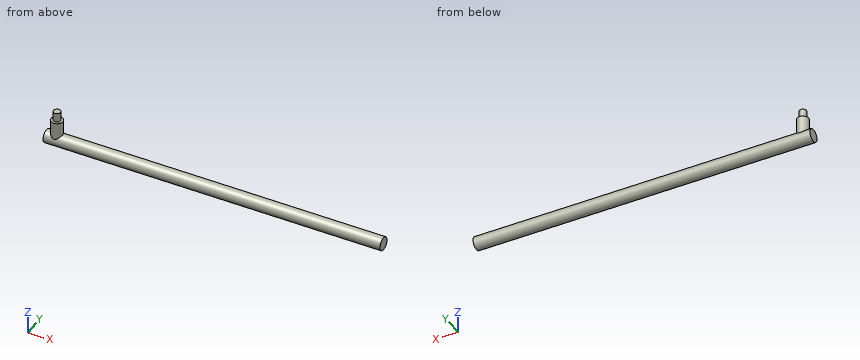
from build123d import *

# Parameters (mm, degrees)
F0_R     = 27.085871
F1_DEPTH = 1397
F2_R     = 23.906419
F3_DEPTH = 85.852
F4_R     = 14.195516
F5_DEPTH = 38.354


with BuildPart() as f1:
    # F0 (on Right) → F1 (new body)
    with BuildSketch(Plane.YZ):
        Circle(F0_R)
    extrude(amount=F1_DEPTH)

    # F2 (on Top) → F3 (join)
    with BuildSketch(Plane.XY):
        with Locations((43.752357, 0)):
            Circle(F2_R)
    extrude(amount=F3_DEPTH)

    # F4 (on face) → F5 (join)
    with BuildSketch(Plane.XY.offset(85.852)):
        with Locations((43.752357, 0)):
            Circle(F4_R)
    extrude(amount=F5_DEPTH)


solid = f1.part
Could you check a few things on this model? Use its own coordinates, in mm. Round coordinates to 2 decimals unless told otherwise and drop trailing zeros. Order: outer loops, then holes, each group sorted by start corner. A loop starts at its lowest first (then second) coordinate and runs counter-clockwise, first axis right, second up.
Q1. Imagine slicing it at A-A, the plane z = 73.5. List the corners of the cut face in (x, y) for me.
Geometry says:
outline: circle Ø47.81 at (43.75, 0)
Q2. Please list where these lines run through material, in increasing order: probe 1 along Y at (x, z) = (743.5, 3); probe 2 along Y at (x, z) = (848.5, -13); probe 3 along X at (y, z) = (2.5, 65.5).
Geometry says:
probe 1: y = -26.92 to 26.92
probe 2: y = -23.76 to 23.76
probe 3: x = 19.98 to 67.53
Q3. Imagine slicing it at B-B, the plane x = 642.5. List the corners of the cut face in (y, z) for me.
Geometry says:
outline: circle Ø54.17 at (0, 0)
Q4. I'm going to push flat-ended pins straight in: P1, Ø2, axis at y = -21, z = 21.5, coming from the +X side; P2, Ø2, axis at x = 429.5, y = -18, coming from the +Z side; P3, Ø6, axis at x = 504.5, y = 1.5, coming from the -Z side. Where does each tip first touch, or does it pass through?
Geometry says:
P1: stops at x = 56.85
P2: stops at z = 21.09
P3: stops at z = -27.09
